Could you check a few things on this drawing? It's one solid part, dimensions in mm from its lowest x, y, z. A direction names the side the tool comes from. Round coordinates to 2 decimals unless told otherwise and drop trailing zeros. Write each loop counter-clockwise with the first axis right and the second up, starting at its lowest first coordinate (ties: lowest second). Pieces come first, ordered by that corner, then holes. Notation, with made-up numbers: (-39, 54.5) -> (-1, 54.5) arc R18 cw to (-1, 64.5) -> close; hole circle Ø3 at (-6.75, 4.25). An arc over 180 degrees is marked (long way). Answer in a Markdown table with one row per item.
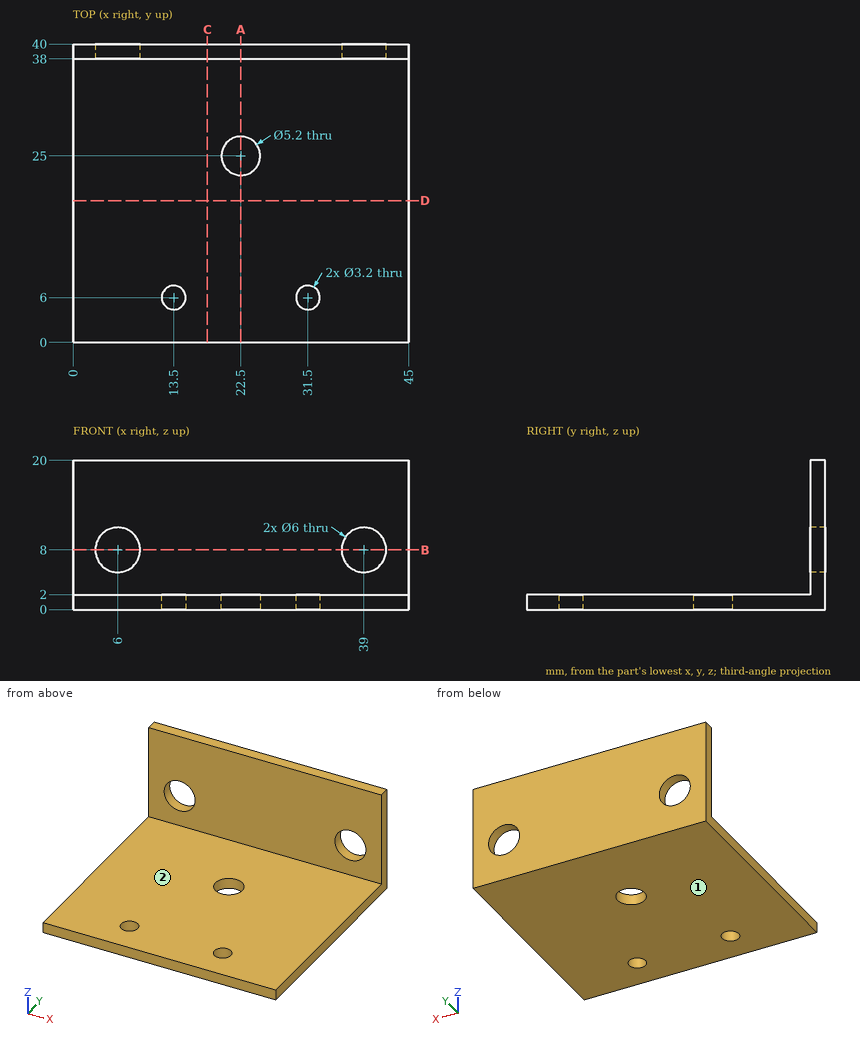
1) I want a section at C-C, the plane x = 18. List the corners of the cut face in (y, z) for me, and give its area (3 significant figures).
Response:
| item | result |
|---|---|
| outline | (0, 0) -> (40, 0) -> (40, 20) -> (38, 20) -> (38, 2) -> (0, 2) -> close |
| area | 116 mm^2 |
2) I want a section at D-D, the plane y = 19. List the corners of the cut face in (x, z) for me, and give its area (3 significant figures).
Response:
| item | result |
|---|---|
| outline | (0, 0) -> (45, 0) -> (45, 2) -> (0, 2) -> close |
| area | 90.0 mm^2 |
3) Which directions (+Z, -Z, +X, -X, +Y, -Y) give clear straight access to the entire face, cutting with the end or side of a thin tool? Please do the marked faces 1 and 2.
Response:
| item | result |
|---|---|
| face 1 | -Z, +X, -X, +Y, -Y |
| face 2 | +Z, +X, -X, -Y |
4) I want a section at A-A, the plane x = 22.5. List the corners of the cut face in (y, z) for me, and give its area (3 significant figures).
Response:
| item | result |
|---|---|
| outline | (0, 0) -> (22.4, 0) -> (22.4, 2) -> (0, 2) -> close; (27.6, 0) -> (40, 0) -> (40, 20) -> (38, 20) -> (38, 2) -> (27.6, 2) -> close |
| area | 106 mm^2 |
5) I want a section at B-B, the plane z = 8. List the corners of the cut face in (x, y) for me, and give its area (3 significant figures).
Response:
| item | result |
|---|---|
| outline | (0, 38) -> (3, 38) -> (3, 40) -> (0, 40) -> close; (9, 38) -> (36, 38) -> (36, 40) -> (9, 40) -> close; (42, 38) -> (45, 38) -> (45, 40) -> (42, 40) -> close |
| area | 66.0 mm^2 |
6) For pin 1 (6 mm diameter, centred on x = 22.5, y = 25, fed in from +Z); pin 2 (8 mm diameter, centred on x = 38.5, y = 7.5, fed in from -Z); pin 3 (5.5 mm diameter, centred on x = 11.5, z = 10, fed in from -Y); pin 4 (3 mm diameter, centred on x = 31.5, y = 6, fed in from +Z), each with a flat end and sliding along its axis, tell me the tip position at first contact or that it passes through.
Response:
| item | result |
|---|---|
| pin 1 | stops at z = 2 |
| pin 2 | stops at z = 0 |
| pin 3 | stops at y = 38 |
| pin 4 | passes through |
7) I need wall thicknesses on line 1 (Z direction, x = 6, y = 38.55); line 2 (Y direction, x = 22.5, z = 0.8); line 3 (Y direction, x = 31.5, z = 0.5). Which ranges of each line are inside material? Lowest first, please. Write a range as [from, to].
Response:
| item | result |
|---|---|
| line 1 | z = [0, 5], [11, 20] |
| line 2 | y = [0, 22.4], [27.6, 40] |
| line 3 | y = [0, 4.4], [7.6, 40] |
